Can you work these out from the model? Positions are in its coordinate system, mm. Face numbers are marked on the shaded views. A direction names the side the tool comes from. Give positions to 0.01 mm unless a question says otherwise; leave off trailing zeros. Write each loop counter-clockwise with the first axis right and the second up, starting at its lowest first coordinate (ties: lowest second). Pieces come first, ordered by that corner, then holes. Notation, with made-up numbers: (74.5, 63) -> (124.5, 63) arc R19 cw to (124.5, 85) -> close; hole circle Ø4 at (-4.75, 43). An arc over 180 degrees is marked (long way). One line per item, written item: value.
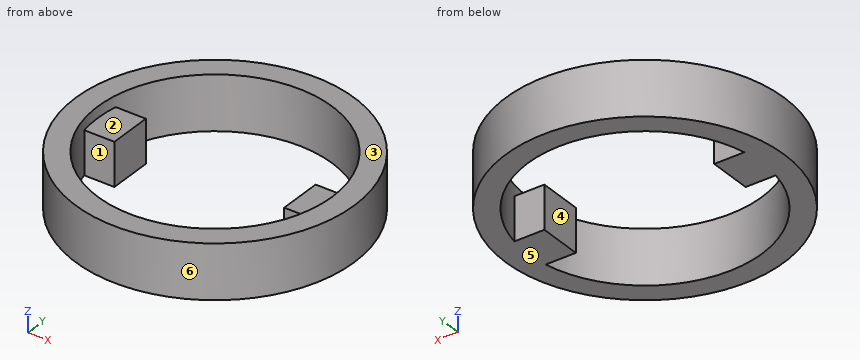
from build123d import *

# Parameters (mm, degrees)
SKETCH_1_R      = 12.55
SKETCH_1_R_2    = 10.55
EXTRUDE_1_DEPTH = 4.9
SKETCH_2_W      = 3.555672838
SKETCH_2_H      = 3.9
EXTRUDE_2_DEPTH = 3.9


with BuildPart() as part:
    # 草图1 → 拉伸-薄壁1 (new body)
    with BuildSketch(Plane.XY):
        Circle(SKETCH_1_R)
        Circle(SKETCH_1_R_2, mode=Mode.SUBTRACT)
    extrude(amount=EXTRUDE_1_DEPTH)

    # 草图2 → 凸台-拉伸2 (add)
    with BuildSketch(Plane.XY):
        with Locations((-9.432034927, 0)):
            Rectangle(SKETCH_2_W, SKETCH_2_H)
        with Locations((9.432034927, 0)):
            Rectangle(SKETCH_2_W, SKETCH_2_H)
    extrude(amount=EXTRUDE_2_DEPTH)


solid = part.part
1) If we section it at C-C (x = 0): Write out the boundary of the cut face in (y, z), and give its area (3 significant figures).
Answer list:
outline: (-12.55, 0) -> (-10.55, 0) -> (-10.55, 4.9) -> (-12.55, 4.9) -> close; (10.55, 0) -> (12.55, 0) -> (12.55, 4.9) -> (10.55, 4.9) -> close
area: 19.6 mm^2
2) I need wall thicknesses on L1, parallel to Y at x = 0, z = 1.95; L2, parallel to X at y = -6.5, z = 0.6; L3, parallel to X at y = -6.75, z = 4.1. Which ranges of each line are inside material? Lowest first, please.
Answer list:
L1: y = -12.55 to -10.55, 10.55 to 12.55
L2: x = -10.74 to -8.31, 8.31 to 10.74
L3: x = -10.58 to -8.11, 8.11 to 10.58
3) If we section it at B-B (z = 1.2): Write out the boundary of the cut face in (x, y), and give its area (3 significant figures).
Answer list:
outline: circle Ø25.1 at (0, 0); hole (-10.37, -1.95) arc R10.55 ccw to (10.37, -1.95) -> (7.65, -1.95) -> (7.65, 1.95) -> (10.37, 1.95) arc R10.55 ccw to (-10.37, 1.95) -> (-7.65, 1.95) -> (-7.65, -1.95) -> close
area: 167 mm^2
4) We'd pull the mould along Y, two halves only. Please class the marked faces 4, 5 and 6: released by +Y, released by -Y, zero draft, split by the parting line, or undercut.
Answer list:
face 4: undercut
face 5: zero draft
face 6: split by the parting line
5) If we section it at D-D (x = -9): Write out the boundary of the cut face in (y, z), and give its area (3 significant figures).
Answer list:
outline: (-8.75, 0) -> (-5.5, 0) -> (-5.5, 4.9) -> (-8.75, 4.9) -> close; (-1.95, 0) -> (1.95, 0) -> (1.95, 3.9) -> (-1.95, 3.9) -> close; (5.5, 0) -> (8.75, 0) -> (8.75, 4.9) -> (5.5, 4.9) -> close
area: 47.0 mm^2
6) Will these pins go through, and if not, where does the flat tip stop? pin 1 (0.9 mm diameter, centred on x = 9.5, y = 0, fed in from +Z); pin 2 (0.8 mm diameter, centred on x = -9.5, z = 2.5, fed in from -Y); pin 3 (1.4 mm diameter, centred on x = 9, z = 1, fed in from -Y).
Answer list:
pin 1: stops at z = 3.9
pin 2: stops at y = -8.64
pin 3: stops at y = -9.41
7) If we section it at A-A (y = 0): Write out the boundary of the cut face in (x, z), and give its area (3 significant figures).
Answer list:
outline: (-12.55, 0) -> (-7.65, 0) -> (-7.65, 3.9) -> (-10.55, 3.9) -> (-10.55, 4.9) -> (-12.55, 4.9) -> close; (7.65, 0) -> (12.55, 0) -> (12.55, 4.9) -> (10.55, 4.9) -> (10.55, 3.9) -> (7.65, 3.9) -> close
area: 42.2 mm^2
8) For the marked faces 1, 2 and 3, which set-ups out of +Z, -Z, +X, -X, +Y, -Y let a thin tool reach every point of the face, with its end or its side?
Answer list:
face 1: +Z, -Z
face 2: +Z
face 3: +Z, +X, -X, +Y, -Y
